```python
from build123d import *

# Parameters (mm, degrees)
SKETCH1_W           = 104.999999998
SKETCH1_H           = 61.999999997
SKETCH1_W_2         = 102
SKETCH1_H_2         = 59
BOSS_EXTRUDE1_DEPTH = 2
SKETCH1_2_W         = 102
SKETCH1_2_H         = 59
BOSS_EXTRUDE2_DEPTH = 2
FILLET1_R           = 2


with BuildPart() as part:
    # Sketch1 → Boss-Extrude1 (new body)
    with BuildSketch(Plane(origin=(0, 0, 0), x_dir=(1, 0, 0), z_dir=(0, 1, 0))):
        with Locations((3.062796012, -2.779331445)):
            Rectangle(SKETCH1_W, SKETCH1_H)
        with Locations((3.062796013, -2.779331447)):
            Rectangle(SKETCH1_W_2, SKETCH1_H_2, mode=Mode.SUBTRACT)
    extrude(amount=BOSS_EXTRUDE1_DEPTH)

    # Sketch1<2> → Boss-Extrude2 (add)
    with BuildSketch(Plane(origin=(0, 0, 0), x_dir=(1, 0, 0), z_dir=(0, 1, 0))):
        with Locations((3.062796013, -2.779331447)):
            Rectangle(SKETCH1_2_W, SKETCH1_2_H)
    extrude(amount=BOSS_EXTRUDE2_DEPTH)

    # Fillet1
    fillet1_edges = [part.edges().sort_by_distance(p)[0] for p in [
        (3.062796012, 0, 33.779331444),
        (55.562796011, 0, 2.779331445),
        (3.062796012, 0, -28.220668553),
        (-49.437203987, 0, 2.779331445),
    ]]
    fillet(fillet1_edges, radius=FILLET1_R - 0.0001)  # a hair under: the kernel refuses the full size


solid = part.part
```
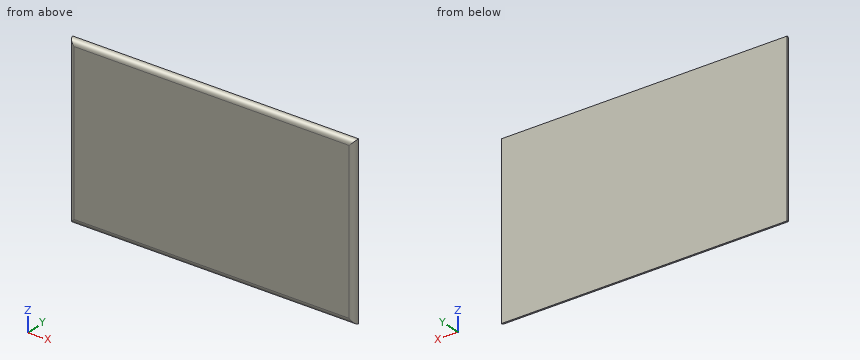
The listing builds one solid part. Answer for the finished solid, in the listing's coordinates (mm). Give positions to 0.01 mm unless a question says otherwise; leave off trailing zeros. Order: outer loops, then holes, each group sorted by start corner. A loop starts at its lowest first (then second) coordinate and runs counter-clockwise, first axis right, second up. Notation, with made-up numbers: M 10,0 L 60,0 A26 cw 60,37 Z; hole C 45.5,25.25 d8. An arc over 180 degrees is marked long. Put each result on its own line as item: value. Start each with the question number.
Item 1: The part is cut by section A-A, the plane y = 0.3. Determine the outline of the cut face in (x, z), and give its area (3 significant figures).
Item 2: Find the intervals of material crossed by line 1 along Z through (x, y) = (33, 1.8); line 2 along Z through (x, y) = (32.5, 1.55); line 3 along X through (y, z) = (0.35, 22.5), in increasing order.
Item 3: A flat-ended cylindrical pin translates along its axis: P1, Ø1, axis at x = 19, y = 1, coming from the -Z side. Find the tip coordinate at first contact, or state that the pin passes through.
Answer key:
1. outline: M -48.49,-27.27 L 54.62,-27.27 L 54.62,32.83 L -48.49,32.83 Z
1. area: 6,200 mm²
2. line 1: z = -28.21 to 33.77
2. line 2: z = -28.17 to 33.73
2. line 3: x = -48.57 to 54.69
3. P1: stops at z = -28.16
